Print and shaded views of the part. All mm, measured from the part's lowest x, y and z. Round coordinates to 2 decimals unless told otherwise and drop trailing zeros. Loops run counter-clockwise (first coordinate to the right, second up) from the corner with the lowest first, then second, coordinate; pieces in that order, holes last. Notation, with made-up numbers: (67, -29.5) -> (73, -29.5) arc R25 ccw to (73, 5.5) -> close; hole circle Ø11 at (69, -31.75). An arc over 180 degrees is marked (long way). Answer as CSV lines item,"result".
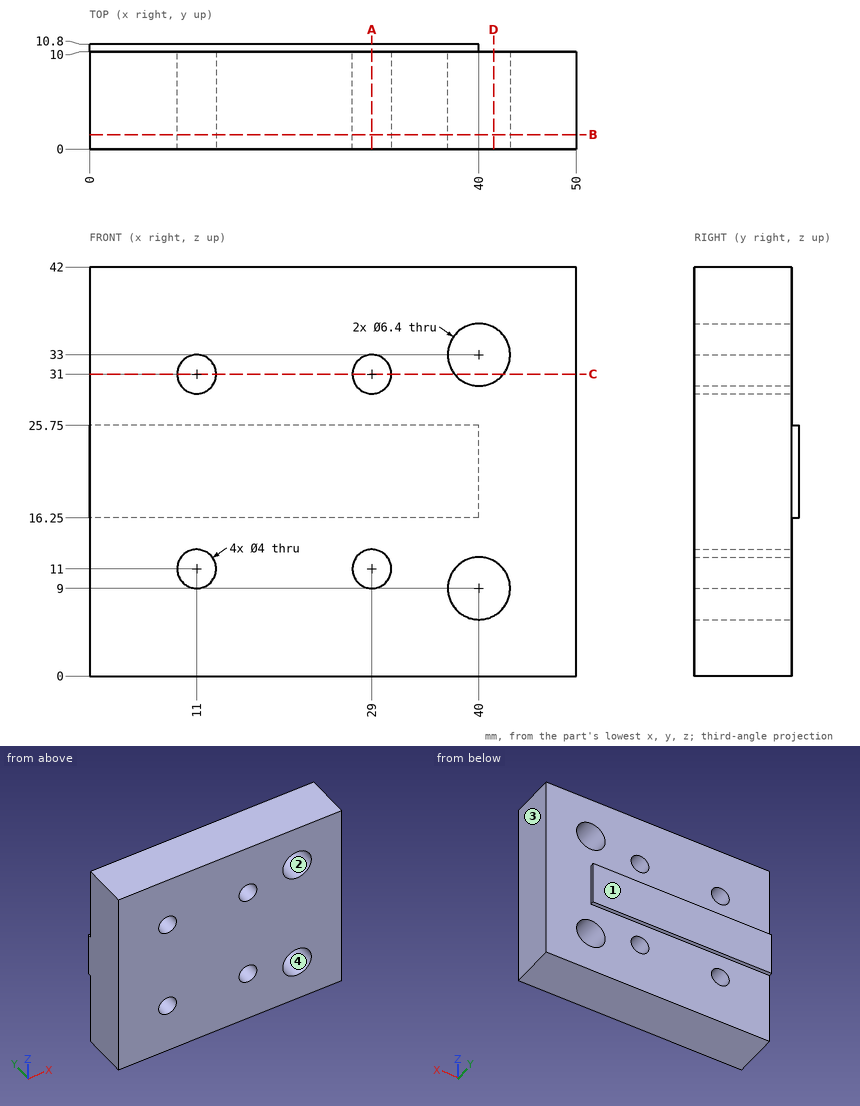
Q1. Drop flat-ended pins along their axis: pin 1 Ø3 at (x, z) = (11, 31) entering from +Y; pin 2 Ø2 at (x, z) = (28, 27) entering from +Y. Give the stop position or say it passes through.
Results:
pin 1,"through"
pin 2,"y = 10"
Q2. Slice it at D-D, the plane x = 41.5. Give the cut face in (y, z).
Results:
outline,"(0, 0) -> (10, 0) -> (10, 6.17) -> (0, 6.17) -> close; (0, 11.83) -> (10, 11.83) -> (10, 30.17) -> (0, 30.17) -> close; (0, 35.83) -> (10, 35.83) -> (10, 42) -> (0, 42) -> close"
Q3. Probe L1, parallel to Z at x = 40, y = 6; L2, parallel to Z at x = 11, y = 5.75; L3, parallel to X at y = 5, z = 32. List the from-to ranges inside material, lowest first. Write a range as [from, to].
Results:
L1,"[0, 5.8], [12.2, 29.8], [36.2, 42]"
L2,"[0, 9], [13, 29], [33, 42]"
L3,"[0, 9.27], [12.73, 27.27], [30.73, 36.96], [43.04, 50]"
Q4. Two-plate mould, pull along X, no slides. Class the marked faces 1, 2, 3 and 4: pulls with the +X half, pulls with the -X half, needs draft (parallel to the pull), parting line crosses it, or undercut.
Results:
face 1,"needs draft"
face 2,"undercut"
face 3,"pulls with the +X half"
face 4,"undercut"
Q5. Slice it at B-B, the plane y = 1.5. Give the cut face in (x, z), and give its area (3 significant figures).
Results:
outline,"(0, 0) -> (50, 0) -> (50, 42) -> (0, 42) -> close; hole circle Ø4 at (11, 11); hole circle Ø4 at (11, 31); hole circle Ø4 at (29, 11); hole circle Ø4 at (29, 31); hole circle Ø6.4 at (40, 9); hole circle Ø6.4 at (40, 33)"
area,"1,990 mm2"
Q6. Slice it at A-A, the plane x = 29. Give the cut face in (y, z), and give its area (3 significant figures).
Results:
outline,"(0, 0) -> (10, 0) -> (10, 9) -> (0, 9) -> close; (0, 13) -> (10, 13) -> (10, 16.25) -> (10.8, 16.25) -> (10.8, 25.75) -> (10, 25.75) -> (10, 29) -> (0, 29) -> close; (0, 33) -> (10, 33) -> (10, 42) -> (0, 42) -> close"
area,"348 mm2"
Q7. Slice it at C-C, the plane z = 31. Give the cut face in (x, y).
Results:
outline,"(0, 0) -> (9, 0) -> (9, 10) -> (0, 10) -> close; (13, 0) -> (27, 0) -> (27, 10) -> (13, 10) -> close; (31, 0) -> (37.5, 0) -> (37.5, 10) -> (31, 10) -> close; (42.5, 0) -> (50, 0) -> (50, 10) -> (42.5, 10) -> close"
